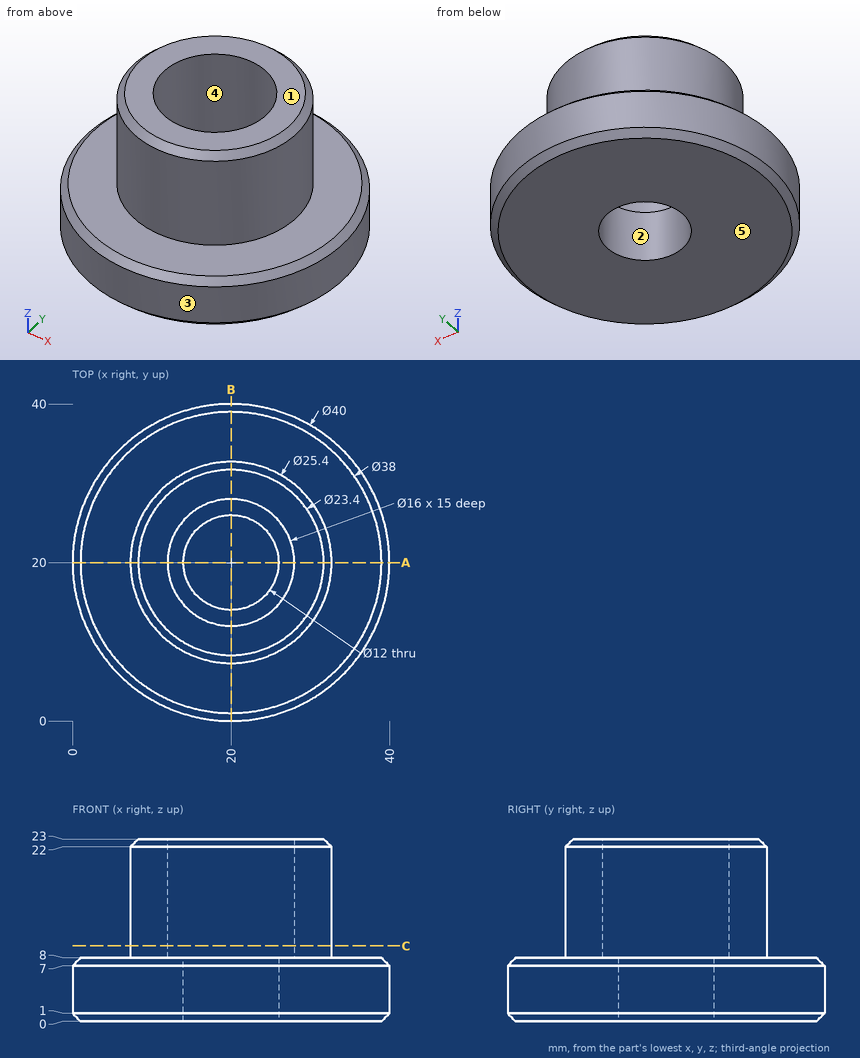
Design review of the part shown in the three views and the two pictorial views. Dimensions are in mm from the part's minimum x, y and z. A direction names the side the tool comes from. Give positions to 0.01 mm unless a question says otherwise; leave off trailing zeros. Loops run counter-clockwise (first coordinate to the right, second up) from the corner with the lowest first, then second, coordinate; pieces in that order, holes last. Notation, with made-up numbers: (45.5, 64) - (78.5, 64) arc R26 ccw to (78.5, 87) - close; hole circle Ø2 at (-14, 38). An arc over 180 degrees is marked (long way). Write item = value, one per line.
1) Take a section at A-A on y = 20. State the section outline as (x, z) points.
Result sheet:
outline = (0, 1) - (1, 0) - (14, 0) - (14, 8) - (12, 8) - (12, 23) - (8.3, 23) - (7.3, 22) - (7.3, 8) - (1, 8) - (0, 7) - close; (26, 0) - (39, 0) - (40, 1) - (40, 7) - (39, 8) - (32.7, 8) - (32.7, 22) - (31.7, 23) - (28, 23) - (28, 8) - (26, 8) - close
2) Take a section at C-C on z = 9.5. State the section outline as (x, y) points.
Result sheet:
outline = circle Ø25.4 at (20, 20); hole circle Ø16 at (20, 20)
3) Clearance check with flat-ended pins moving along their axes: pin 1 Ø10 at (x, z) = (17.5, 15) entering from -Y; pin 2 Ø1 at (y, z) = (17.5, 13) entering from -X; pin 3 Ø5 at (x, y) = (22.5, 20.5) entering from +Z; pin 4 Ø3 at (x, z) = (17.5, 6.5) entering from +Y (3 decimals). State where each tip first meets the part, or that it passes through.
Result sheet:
pin_1 = 7.3
pin_2 = 7.46
pin_3 = through
pin_4 = 39.975
4) Draft analysis for pull direction Y (two halves, no side actions). For the marked faces 1, 2 and 3, state which applies: +Y half, -Y half, draft (parallel to the pull), parting line (faces both ways), or undercut.
Result sheet:
face_1 = draft
face_2 = undercut
face_3 = parting line
5) To check wall thickness, follow line 1 (Y direction, x = 20, z = 13.5); line 2 (Y direction, x = 20, z = 6); line 3 (Z direction, x = 31.5, y = 9.5). State the ranges of each line that lie inside material, in increasing order.
Result sheet:
line_1 = 7.3 to 12, 28 to 32.7
line_2 = 0 to 14, 26 to 40
line_3 = 0 to 8
6) Tool access review of the marked faces 4 and 5: name each direction out of +Z, -Z, +X, -X, +Y, -Y from which nothing blocks a thin tool from reaching the whole face with its end or side.
Result sheet:
face_4 = +Z
face_5 = -Z, +X, -X, +Y, -Y
